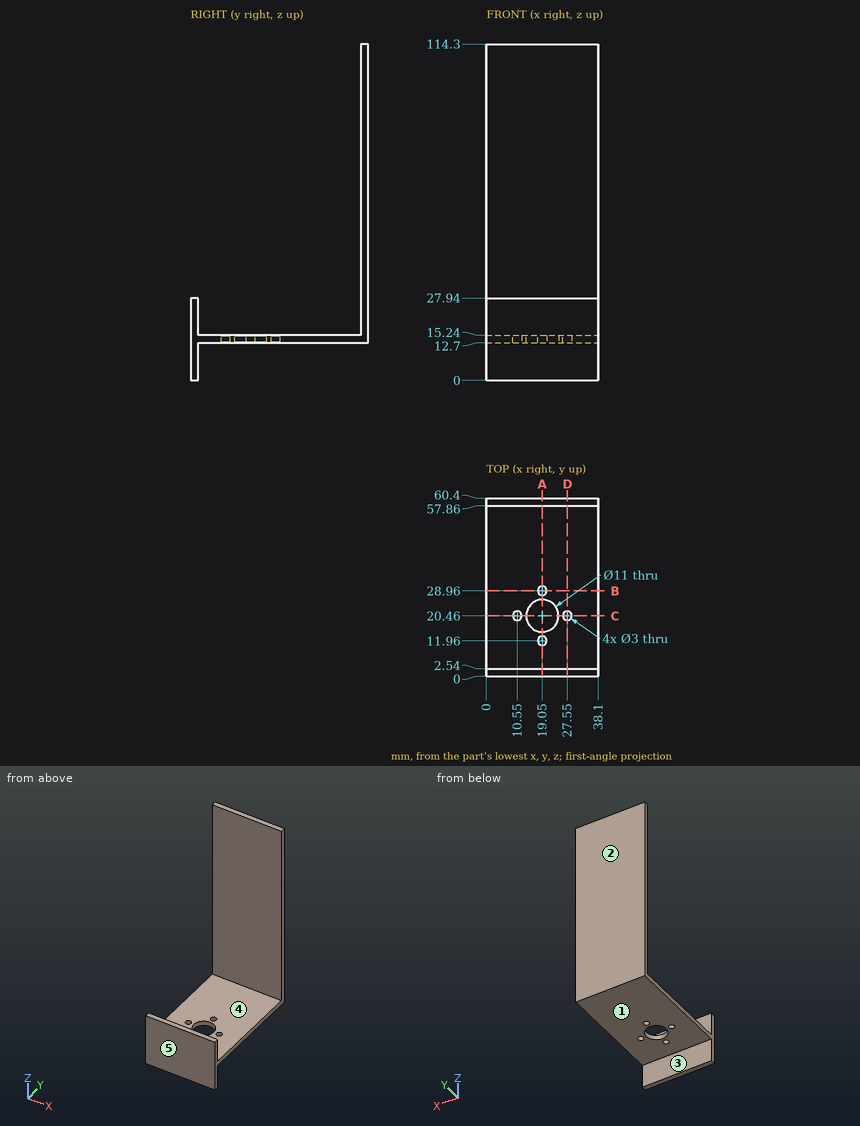
Check sheet for the drawn part. Datum: minimum x, y, z corner. Units: mm. A direction names the side the tool comes from. Round coordinates to 2 decimals unless told otherwise and drop trailing zeros. Order: outer loops, then holes, each group sorted by start corner. A loop starts at its lowest first (then second) coordinate and runs counter-clockwise, first axis right, second up. Notation, with made-up numbers: (42.5, 84) - (87.5, 84) arc R17 cw to (87.5, 106) - close; hole circle Ø3 at (-7.5, -2.75). An arc over 180 degrees is marked (long way). Use a Markdown table: item, result. Add a question column.
(1) Sectioned sample at D-D, the plane x = 27.55. Enter the section's corners in (y, z), and give its area (3 significant figures).
(2) Release check for a two-part mould opening along Y. For the marked faces 3, 4 and 5 record: pulls with the +Y half, pulls with the -Y half, needs draft (parallel to the pull), parting line crosses it, or undercut.
(3) Depth check by flat-ended pin: pin 1 (11.5 mm diameter, centred on x = 16.5, y = 41.5, fed in from +Z); pin 2 (2.5 mm diameter, centred on x = 19.05, y = 28.96, fed in from +Z); pin 3 (3 mm diameter, centred on x = 6, y = 51, fed in from -Z); pin 4 (6 mm diameter, centred on x = 5, z = 101, fed in from -Y). Enter the tip coordinate at first touch or a pass-through.
(4) Material ranges on line 1 along Y through (x, z) = (19.05, 14); line 2 along X through (y, z) = (20, 13); line 3 along Y through (x, z) = (23, 23.5), recorded low to high. Write a range as [from, to].
(5) Sectioned sample at C-C, the plane y = 20.46. Enter the section's corners in (x, z).
(6) Sectioned sample at A-A, the plane x = 19.05. Enter the section's corners in (y, z).
(7) Sectioned sample at B-B, the plane y = 28.96. Enter the section's corners in (x, z), and give its area (3 significant figures).
(8) Tool access check on the marked faces 1 and 2. Record the directions out of +Z, -Z, +X, -X, +Y, -Y that give a thin tool (end or side, any length) a straight path to the whole face; none if there is none.
Answers below:
| question | item | result |
|---|---|---|
| 1 | outline | (0, 0) - (2.54, 0) - (2.54, 12.7) - (18.96, 12.7) - (18.96, 15.24) - (2.54, 15.24) - (2.54, 27.94) - (0, 27.94) - close; (21.96, 12.7) - (60.4, 12.7) - (60.4, 114.3) - (57.86, 114.3) - (57.86, 15.24) - (21.96, 15.24) - close |
| 1 | area | 462 mm² |
| 2 | face 3 | pulls with the +Y half |
| 2 | face 4 | undercut |
| 2 | face 5 | pulls with the -Y half |
| 3 | pin 1 | z = 15.24 |
| 3 | pin 2 | through |
| 3 | pin 3 | z = 12.7 |
| 3 | pin 4 | y = 57.86 |
| 4 | line 1 | [0, 10.46], [13.46, 14.96], [25.96, 27.46], [30.46, 60.4] |
| 4 | line 2 | [0, 9.12], [11.98, 13.57], [24.53, 26.12], [28.98, 38.1] |
| 4 | line 3 | [0, 2.54], [57.86, 60.4] |
| 5 | outline | (0, 12.7) - (9.05, 12.7) - (9.05, 15.24) - (0, 15.24) - close; (12.05, 12.7) - (13.55, 12.7) - (13.55, 15.24) - (12.05, 15.24) - close; (24.55, 12.7) - (26.05, 12.7) - (26.05, 15.24) - (24.55, 15.24) - close; (29.05, 12.7) - (38.1, 12.7) - (38.1, 15.24) - (29.05, 15.24) - close |
| 6 | outline | (0, 0) - (2.54, 0) - (2.54, 12.7) - (10.46, 12.7) - (10.46, 15.24) - (2.54, 15.24) - (2.54, 27.94) - (0, 27.94) - close; (13.46, 12.7) - (14.96, 12.7) - (14.96, 15.24) - (13.46, 15.24) - close; (25.96, 12.7) - (27.46, 12.7) - (27.46, 15.24) - (25.96, 15.24) - close; (30.46, 12.7) - (60.4, 12.7) - (60.4, 114.3) - (57.86, 114.3) - (57.86, 15.24) - (30.46, 15.24) - close |
| 7 | outline | (0, 12.7) - (17.55, 12.7) - (17.55, 15.24) - (0, 15.24) - close; (20.55, 12.7) - (38.1, 12.7) - (38.1, 15.24) - (20.55, 15.24) - close |
| 7 | area | 89.2 mm² |
| 8 | face 1 | -Z, +X, -X, +Y |
| 8 | face 2 | +Z, -Z, +X, -X, +Y |
